Autodesk Inventor part; units mm, degrees
ref_plane "YZ Plane" through (0, 0, 0) normal (1, 0, 0) x (0, 1, 0)
ref_plane "XZ Plane" through (0, 0, 0) normal (0, 1, 0) x (-1, 0, 0)
ref_plane "XY Plane" through (0, 0, 0) normal (0, 0, 1) x (1, 0, 0)
sketch "Sketch1" plane through (0, 0, 0) normal (0, 1, 0) x (-1, 0, 0)
  line L0 (0, 0) -> (-28, 0)
  line L1 (-28, 0) -> (-28, 28)
  line L2 (-28, 28) -> (0, 28)
  line L3 (0, 28) -> (0, 0)
  dimension "d0" = 28
  dimension "d1" = 28
extrude "Extrusion1" add sketch "Sketch1" along normal blind 4
sketch "Sketch2" plane through (0, 0, 0) normal (0, -1, 0) x (1, 0, 0)
  line L0 (0, 28) -> (28, 28)
  line L1 (14, 28) -> (19, 28)
  line L2 (19, 28) -> (19, 24)
  line L3 (19, 24) -> (9, 24)
  line L4 (9, 24) -> (9, 28)
  point P0 (0, 0)
  dimension "d6" = 5
  dimension "d7" = 4
  dimension "d8" = 10
extrude "Extrusion2" add sketch "Sketch2" along normal blind 8
properties part number "Schemo lcd"
Read the model definition and answer for the solid it produces. Units are mm, in the model's axes. A direction names the side the tool comes from. Coordinates: 2 decimals unless noted, no trailing zeros. Order: outer loops, then holes, each group sorted by start corner. A loop starts at its lowest first (then second) coordinate and runs counter-clockwise, first axis right, second up. Notation, with made-up numbers: (-4.5, 33) - (51.5, 33) arc R20 ccw to (51.5, 61) - close; hole circle Ø9 at (-17.75, 33). An arc over 180 degrees is marked (long way). Use one line per item in the form item = value.
(1) Given pin 1 Ø5 at (x, y) = (21, -6.5) entering from +Z; pin 2 Ø1.2 at (y, z) = (-2, 26) entering from -X; pin 3 Ø1 at (x, z) = (7.5, 12.5) entering from -Y; pin 4 Ø4 at (x, y) = (14, -5) entering from -Z, each flat-ended and moving along its own axis, determine where each tip first touches the part or whether it passes through.
Computed values:
pin_1 = 28
pin_2 = 9
pin_3 = 0
pin_4 = 24
(2) For a pull along Y with two mould halves and no side action, classify faces 1 (the face through (14, 4, 14)), 2 (the face through (14, -8, 26)), 3 (the face through (0, 2, 14)) as pulls with the +Y half, pulls with the -Y half, needs draft (parallel to the pull), parting line crosses it, or undercut.
Computed values:
face_1 = pulls with the +Y half
face_2 = pulls with the -Y half
face_3 = needs draft
(3) Straight lines are drawn through the part: L1, parallel to Y at x = 10, z = 10.75; L2, parallel to X at y = -6.75, z = 26; L3, parallel to Z at x = 12.5, y = -1.5. For each, find the intervals that lie inside material, in ascending order.
Computed values:
L1 = 0 to 4
L2 = 9 to 19
L3 = 24 to 28
(4) Section C-C, the plane y = -6.75 is taken. Give the vertices of the cut face in (x, z).
Computed values:
outline = (9, 24) - (19, 24) - (19, 28) - (9, 28) - close
(5) Which of the six approach directions +Z, -Z, +X, -X, +Y, -Y give full straight-line access (tool end or side, diameter ignored) to faces 4 (the face through (14, -1, 28)), 5 (the face through (9, -4, 26)), 6 (the face through (19, -4, 26)), 7 (the face through (14, -4, 24)), 8 (the face through (28, 2, 14))?
Computed values:
face_4 = +Z, +X, -X, +Y, -Y
face_5 = +Z, -Z, -X, -Y
face_6 = +Z, -Z, +X, -Y
face_7 = -Z, +X, -X, -Y
face_8 = +Z, -Z, +X, +Y, -Y
(6) Section A-A, the plane z = 24.75 is taken. Give the vertices of the cut face in (x, y), then the cut area to 3 significant figures.
Computed values:
outline = (0, 0) - (9, 0) - (9, -8) - (19, -8) - (19, 0) - (28, 0) - (28, 4) - (0, 4) - close
area = 192 mm²
(7) Section D-D, the plane x = 8 is taken. Give the vertices of the cut face in (y, z).
Computed values:
outline = (0, 0) - (4, 0) - (4, 28) - (0, 28) - close
(8) Section B-B, the plane x = 14.5 is taken. Give the vertices of the cut face in (y, z).
Computed values:
outline = (-8, 24) - (0, 24) - (0, 0) - (4, 0) - (4, 28) - (-8, 28) - close
